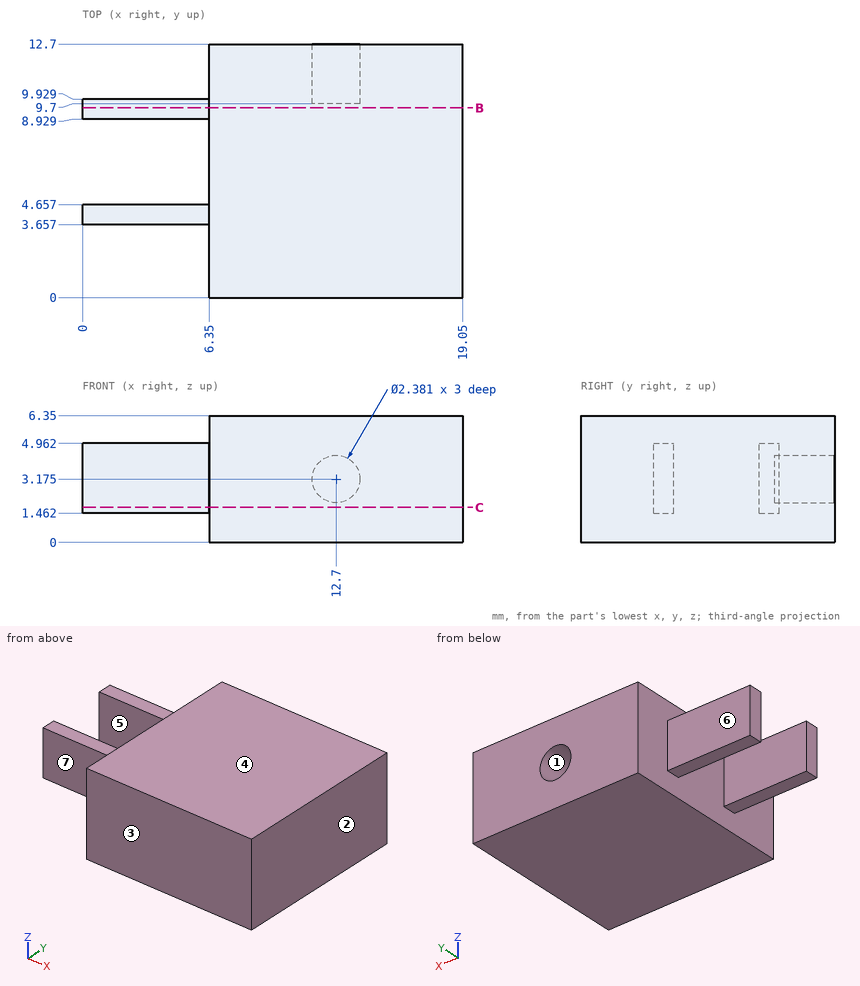
Here's the drawing with two shaded views (mm, measured from the low corner). I have some questions. A direction names the side the tool comes from. Coordinates: 2 decimals unless noted, no trailing zeros. Write each loop counter-clockwise with the first axis right and the second up, starting at its lowest first coordinate (ties: lowest second). Pieces come first, ordered by that corner, then holes. Notation, with made-up numbers: M 77.25,43.5 L 127.25,43.5 A23 cw 127.25,82.5 Z; hole C -35,77.25 d4. An arc over 180 degrees is marked long. Answer as CSV lines item,"result". Start each with the question number.
1) For P1, Ø3, axis at y = 1.5, z = 4, coming from the -X side; P2, Ø1.1, axis at x = 2, y = 9.5, coming from the -Z side; P3, Ø2, axis at x = 12.7, z = 3.175, coming from the -Y side; P4, Ø1.1, axis at x = 4, y = 9.5, coming from the +Z side, each with a flat end and sliding along its axis, tell me the tip position at first contact or that it passes through.
2) For the marked faces 4, 5, 6 and 7, which set-ups out of +Z, -Z, +X, -X, +Y, -Y let a thin tool reach every point of the face, with its end or its side?
3) I want a section at B-B, the plane y = 9.5. Please give me the cut outline in (x, z).
4) We'd pull the mould along X, two halves only. Please class the marked faces 1, 2 and 3: +X half, -X half, draft (parallel to the pull), parting line (faces both ways), or undercut.
5) Please list where these lines run through material, in increasing order: line 1 (Y direction, x = 5.5, z = 2.75); line 2 (X direction, y = 4, z = 1); line 3 (Z direction, x = 1, y = 4). Write a range as from..to.
6) I want a section at C-C, the plane z = 1.75. Please give me the cut outline in (x, y).
Data:
1,P1,"stops at x = 6.35"
1,P2,"stops at z = 1.46"
1,P3,"stops at y = 0"
1,P4,"stops at z = 4.96"
2,face 4,"+Z, +X, -X, +Y, -Y"
2,face 5,"+Z, -Z, -X"
2,face 6,"+Z, -Z, -X, +Y"
2,face 7,"+Z, -Z, -X, -Y"
3,outline,"M 0,1.46 L 6.35,1.46 L 6.35,0 L 19.05,0 L 19.05,6.35 L 6.35,6.35 L 6.35,4.96 L 0,4.96 Z"
4,face 1,"undercut"
4,face 2,"+X half"
4,face 3,"draft"
5,line 1,"y = 3.66..4.66, 8.93..9.93"
5,line 2,"x = 6.35..19.05"
5,line 3,"z = 1.46..4.96"
6,outline,"M 0,3.66 L 6.35,3.66 L 6.35,0 L 19.05,0 L 19.05,12.7 L 6.35,12.7 L 6.35,9.93 L 0,9.93 L 0,8.93 L 6.35,8.93 L 6.35,4.66 L 0,4.66 Z"
